```python
from build123d import *

# Parameters (mm, degrees)
F0_R     = 9.5631
F1_DEPTH = 2
F3_DEPTH = 0.5
F4_R     = 4
F5_DEPTH = 3.5
F6_R     = 1.2071067812
F7_R     = 2
F8_DEPTH = 2.75
F9_R     = 0.4828427125
F10_R    = 0.4587005769


with BuildPart() as f1:
    # F0 (on Top) → F1 (new body)
    with BuildSketch(Plane.XY):
        Circle(F0_R)
    extrude(amount=F1_DEPTH)

    # F2 (on face) → F3 (cut)
    with BuildSketch(Plane.XY.offset(2)):
        with BuildLine():
            Line((-5.3615504412, 3.1385514695), (-8.9615506499, 3.1385514695))
            Line((-8.9615506499, 3.1385514695), (-8.9615506499, -0.8614485305))
            Line((-8.9615506499, -0.8614485305), (-5.3615504412, -0.8614485305))
            add(Edge.make_bspline(
                [(-5.3615504412, -0.8614485305), (-5.6224469921, -1.1192503233), (-6.0925433919, -1.7012989472), (-6.6913880247, -1.6026951337), (-6.9615501282, -1.56970984)],
                knots=[0, 0, 0, 0, 0.5343034202, 1, 1, 1, 1], degree=3))
            add(Edge.make_bspline(
                [(-6.9615501282, -1.56970984), (-6.8399805695, -1.6500440597), (-6.347646398, -1.9753827537), (-0.9303625125, -6.1475392154), (-0.1936655889, -6.144593355), (0, -6.1438189364)],
                knots=[0, 0, 0, 0, 0.1946474203, 0.7882859605, 1, 1, 1, 1], degree=3))
            add(Edge.make_bspline(
                [(6.9615501282, -1.56970984), (6.8399805695, -1.6500440597), (6.347646398, -1.9753827537), (0.9303625125, -6.1475392154), (0.1936655889, -6.144593355), (0, -6.1438189364)],
                knots=[0, 0, 0, 0, 0.1946474203, 0.7882859605, 1, 1, 1, 1], degree=3))
            add(Edge.make_bspline(
                [(5.3615504412, -0.8614485305), (5.6224469921, -1.1192503233), (6.0925433919, -1.7012989472), (6.6913880247, -1.6026951337), (6.9615501282, -1.56970984)],
                knots=[0, 0, 0, 0, 0.5343034202, 1, 1, 1, 1], degree=3))
            Line((5.3615504412, -0.8614485305), (8.9615506499, -0.8614485305))
            Line((8.9615506499, -0.8614485305), (8.9615506499, 3.1385514695))
            Line((8.9615506499, 3.1385514695), (5.3615504412, 3.1385514695))
            add(Edge.make_bspline(
                [(6.1931497529, 3.8636233108), (6.0443974333, 3.9010068061), (5.670325539, 3.978226764), (5.4715862757, 3.474410976), (5.3615504412, 3.1385514695)],
                knots=[0, 0, 0, 0, 0.4192603681, 1, 1, 1, 1], degree=3))
            Line((6.1931497529, 3.8636233108), (6.1931497529, 4.7969568528))
            add(Edge.make_bspline(
                [(6.1931497529, 4.7969568528), (4.7216724548, 4.9242823231), (2.1318591256, 5.3009462593), (0.6299616116, 6.4122477435), (0, 7.1124638543)],
                knots=[0, 0, 0, 0, 0.5517805711, 1, 1, 1, 1], degree=3))
            add(Edge.make_bspline(
                [(-6.1931497529, 4.7969568528), (-4.7216724548, 4.9242823231), (-2.1318591256, 5.3009462593), (-0.6299616116, 6.4122477435), (0, 7.1124638543)],
                knots=[0, 0, 0, 0, 0.5517805711, 1, 1, 1, 1], degree=3))
            Line((-6.1931497529, 4.7969568528), (-6.1931497529, 3.8636233108))
            add(Edge.make_bspline(
                [(-6.1931497529, 3.8636233108), (-6.0443974333, 3.9010068061), (-5.670325539, 3.978226764), (-5.4715862757, 3.474410976), (-5.3615504412, 3.1385514695)],
                knots=[0, 0, 0, 0, 0.4192603681, 1, 1, 1, 1], degree=3))
        make_face()
        with BuildLine():
            Line((-8.5615506499, -0.4614485305), (-8.5615506499, 2.7385514695))
            Line((-8.5615506499, 2.7385514695), (-4.9470122904, 2.7385514695))
            add(Edge.make_bspline(
                [(-4.9470122904, 2.7385514695), (-5.1446386525, 3.2045990564), (-5.1055478765, 3.9237810781), (-5.5161688277, 4.0677103042), (-5.6931497529, 4.1190395132)],
                knots=[0, 0, 0, 0, 0.6041530811, 1, 1, 1, 1], degree=3))
            Line((-5.6931497529, 4.1190395132), (-5.6931497529, 4.5363726094))
            add(Edge.make_bspline(
                [(-5.6931497529, 4.5363726094), (-4.2737453772, 4.5524962856), (-1.9984707056, 4.9805333611), (-0.5673266444, 5.9968670056), (0, 6.6124638543)],
                knots=[0, 0, 0, 0, 0.5518625842, 1, 1, 1, 1], degree=3))
            add(Edge.make_bspline(
                [(5.6931497529, 4.5363726094), (4.2737453772, 4.5524962856), (1.9984707056, 4.9805333611), (0.5673266444, 5.9968670056), (0, 6.6124638543)],
                knots=[0, 0, 0, 0, 0.5518625842, 1, 1, 1, 1], degree=3))
            Line((5.6931497529, 4.5363726094), (5.6931497529, 4.1190395132))
            add(Edge.make_bspline(
                [(4.9470122904, 2.7385514695), (5.1446386525, 3.2045990564), (5.1055478765, 3.9237810781), (5.5161688277, 4.0677103042), (5.6931497529, 4.1190395132)],
                knots=[0, 0, 0, 0, 0.6041530811, 1, 1, 1, 1], degree=3))
            Line((4.9470122904, 2.7385514695), (8.5615506499, 2.7385514695))
            Line((8.5615506499, 2.7385514695), (8.5615506499, -0.4614485305))
            Line((8.5615506499, -0.4614485305), (4.6812822111, -0.4614485305))
            add(Edge.make_bspline(
                [(4.6812822111, -0.4614485305), (5.1399033686, -1.0753765004), (5.8187100584, -1.7971304682), (5.9548754674, -1.8901632532), (6.0075321235, -1.8750670133)],
                knots=[0, 0, 0, 0, 0.7736948108, 1, 1, 1, 1], degree=3))
            add(Edge.make_bspline(
                [(6.0075321235, -1.8750670133), (3.9265038862, -3.4407765932), (1.0763673429, -5.6147060905), (0.2287364416, -5.721853651), (0, -5.7438189364)],
                knots=[0, 0, 0, 0, 0.7303059463, 1, 1, 1, 1], degree=3))
            add(Edge.make_bspline(
                [(-6.0075321235, -1.8750670133), (-3.9265038862, -3.4407765932), (-1.0763673429, -5.6147060905), (-0.2287364416, -5.721853651), (0, -5.7438189364)],
                knots=[0, 0, 0, 0, 0.7303059463, 1, 1, 1, 1], degree=3))
            add(Edge.make_bspline(
                [(-4.6812822111, -0.4614485305), (-5.1399033686, -1.0753765004), (-5.8187100584, -1.7971304682), (-5.9548754674, -1.8901632532), (-6.0075321235, -1.8750670133)],
                knots=[0, 0, 0, 0, 0.7736948108, 1, 1, 1, 1], degree=3))
            Line((-4.6812822111, -0.4614485305), (-8.5615506499, -0.4614485305))
        make_face(mode=Mode.SUBTRACT)
    extrude(amount=-F3_DEPTH, mode=Mode.SUBTRACT)

    # F4 (on face) → F5 (join)
    with BuildSketch(Plane(origin=(0, 0, 0), x_dir=(1, 0, 0), z_dir=(0, 0, -1))):
        Circle(F4_R)
    extrude(amount=F5_DEPTH)

    # F6
    f6_edges = [f1.edges().sort_by_distance(p)[0] for p in [
        (-9.5631, 0, 0),
    ]]
    fillet(f6_edges, radius=F6_R)

    # F7 (on face) → F8 (join)
    with BuildSketch(Plane(origin=(0, 0, -3.5), x_dir=(1, 0, 0), z_dir=(0, 0, -1))):
        Circle(F7_R)
    extrude(amount=F8_DEPTH)

    # F9
    f9_edges = [f1.edges().sort_by_distance(p)[0] for p in [
        (-2, 0, -6.25),
    ]]
    fillet(f9_edges, radius=F9_R)

    # F10
    f10_edges = [f1.edges().sort_by_distance(p)[0] for p in [
        (-4, 0, -3.5),
    ]]
    fillet(f10_edges, radius=F10_R)


solid = f1.part
```
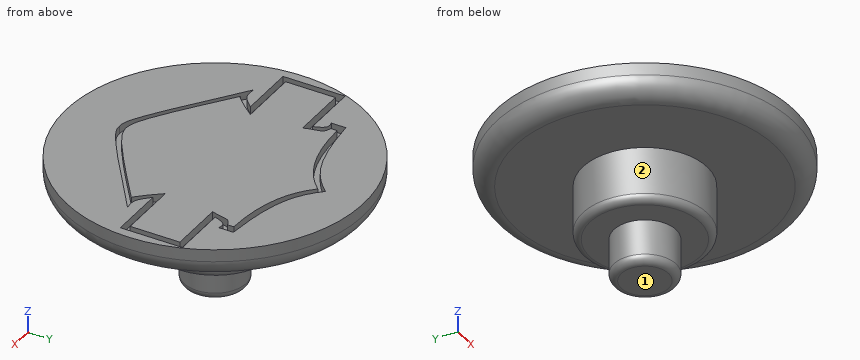
Geometry check sheet. Reference: the model listing, model coordinates, mm. Face numbers are marked on the shaded views. A direction names the side the tool comes from. Coordinates: 2 decimals unless noted, no trailing zeros. Loops run counter-clockwise (first coordinate to the right, second up) from the corner with the lowest first, then second, coordinate; pieces in that order, holes last. Notation, with made-up numbers: (62.25, 60) - (95.25, 60) arc R18 ccw to (95.25, 94) - close; hole circle Ø4 at (-21.75, -5). An arc over 180 degrees is marked (long way). One line per item, written item: value. Start each with the question number.
(1) Tool access check on the marked faces 1 and 2. Record the directions out of +Z, -Z, +X, -X, +Y, -Y that give a thin tool (end or side, any length) a straight path to the whole face; none if there is none.
(2) Cross-section at A-A on y = 0. Enter the section's corners in (x, z).
(3) Depth check by flat-ended pin: P1, Ø2, axis at y = -4, z = -4, coming from the -X side; P2, Ø1, axis at x = -3, y = 0.5, coming from the -Z side; P3, Ø0.6, axis at y = 1.5, z = 2, coming from the +X side. Enter the tip coordinate at first touch or a pass-through.
(4) Cross-section at C-C on z = -2.25. Enter the section's corners in (x, y).
(5) Material ranges on line 1 (Z direction, x = -4.5, y = -1); line 2 (Z direction, x = 2.75, y = -0.75); line 3 (X direction, y = 1.5, z = -2.5), recorded low to high. Write a range as [from, to].
(6) Cross-section at B-B on z = 1.75. Count the separate pieces of the cut face and the enclosed holes in it, plus the area to 3 significant figures.
Results below:
1. face 1: -Z, +X, -X, +Y, -Y
1. face 2: -Z
2. outline: (-9.56, 1.21) arc R1.21 ccw to (-8.36, 0) - (-4, 0) - (-4, -3.04) arc R0.46 ccw to (-3.54, -3.5) - (-2, -3.5) - (-2, -5.77) arc R0.48 ccw to (-1.52, -6.25) - (1.52, -6.25) arc R0.48 ccw to (2, -5.77) - (2, -3.5) - (3.54, -3.5) arc R0.46 ccw to (4, -3.04) - (4, 0) - (8.36, 0) arc R1.21 ccw to (9.56, 1.21) - (9.56, 2) - (8.96, 2) - (8.96, 1.5) - (8.56, 1.5) - (8.56, 2) - (-8.56, 2) - (-8.56, 1.5) - (-8.96, 1.5) - (-8.96, 2) - (-9.56, 2) - close
3. P1: stops at x = -2.14
3. P2: stops at z = -3.5
3. P3: stops at x = 9.49
4. outline: circle Ø8 at (0, 0)
5. line 1: z = [0, 2]
5. line 2: z = [-3.5, 2]
5. line 3: x = [-3.71, 3.71]
6. separate pieces: 2
6. enclosed holes: 1
6. area: 266 mm2
